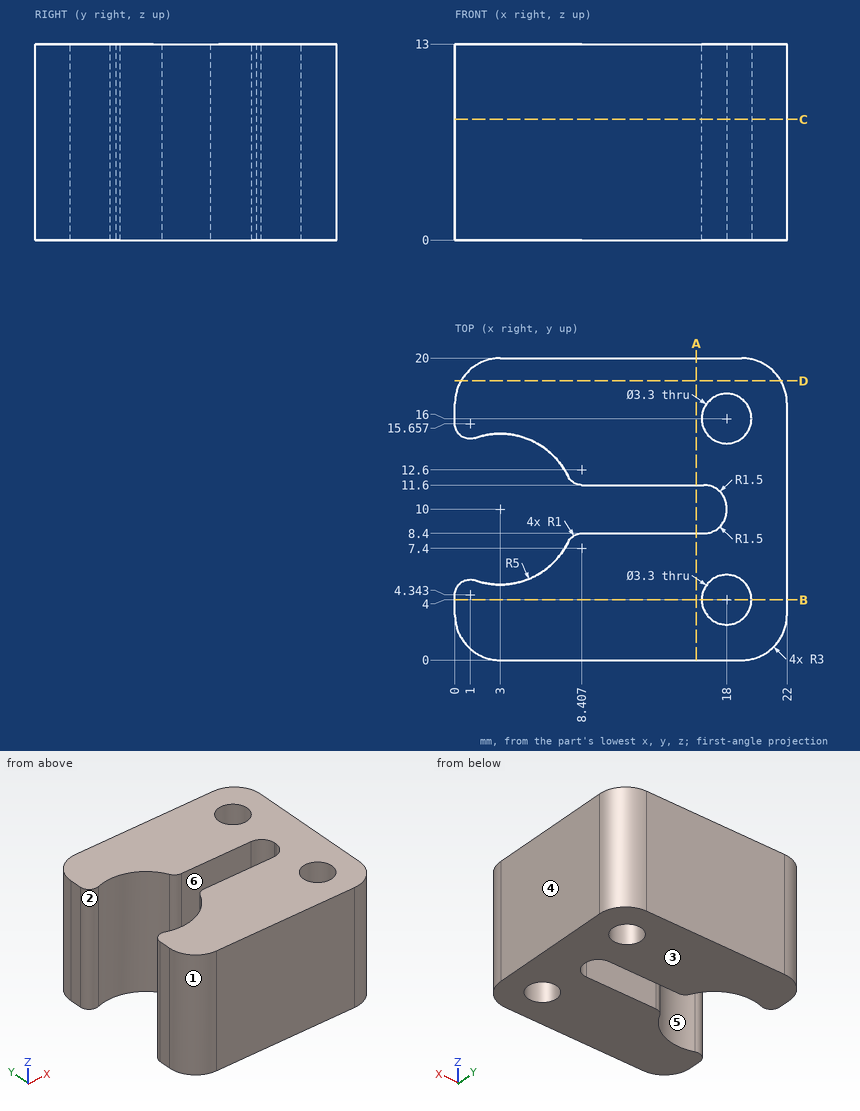
Here's the drawing with two shaded views (mm, measured from the low corner). I have some questions. A direction names the side the tool comes from. Give positions to 0.01 mm unless a question says otherwise; leave off trailing zeros. Loops run counter-clockwise (first coordinate to the right, second up) from the corner with the lowest first, then second, coordinate; pieces in that order, holes last. Notation, with made-up numbers: (-20, 68.5) - (21, 68.5) arc R37 cw to (21, 107.5) - close; hole circle Ø5 at (8, 79.25). An arc over 180 degrees is marked (long way). Answer in a Markdown table with one row per item. Add a question column.
Q1. If we section it at B-B (y = 4): List the corners of the cut face in (x, z) for me, plus the area to 3 significant figures.
Q2. For pin 1 (6 mm diameter, centred on y = 9.5, z = 6.5, fed in from -X); pin 2 (2.5 mm diameter, centred on x = 18, y = 16, fed in from +Z), each with a flat end and sliding along its axis, tell me the tip position at first contact or that it passes through.
Q3. Please list where these lines run through material, in increasing order: L1, parallel to Y at x = 14, z = 9.5; L2, parallel to Y at x = 4.75, z = 12.25 (1 decimal); L3, parallel to Y at x = 16.75, z = 10.5 (1 decimal). Write a range as from..to.
Q4. We'd pull the mould along X, two halves only. Please class the marked faces 1, 2 and 3: +X half, -X half, draft (parallel to the pull), parting line (faces both ways), or undercut.
Q5. If we section it at C-C (z = 8): List the corners of the cut face in (x, y) for me, plus the area to 3 significant figures.
Q6. Which directions (+Z, -Z, +X, -X, +Y, -Y) give clear straight access to the entire face, cutting with the end or side of a thin tool? Please do the marked faces 4, 5 and 6.
Q7. If we section it at D-D (y = 18.5): List the corners of the cut face in (x, z) for me.
Q8. If we section it at A-A (x = 16): List the corners of the cut face in (y, z) for me.
The answers:
| question | item | result |
|---|---|---|
| 1 | outline | (0, 0) - (16.35, 0) - (16.35, 13) - (0, 13) - close; (19.65, 0) - (22, 0) - (22, 13) - (19.65, 13) - close |
| 1 | area | 243 mm^2 |
| 2 | pin 1 | stops at x = 6.57 |
| 2 | pin 2 | passes through |
| 3 | L1 | y = 0..8.4, 11.6..20 |
| 3 | L2 | y = 0..5.3, 14.7..20 |
| 3 | L3 | y = 0..2.9, 5.1..8.4, 11.6..14.9, 17.1..20 |
| 4 | face 1 | -X half |
| 4 | face 2 | undercut |
| 4 | face 3 | draft |
| 5 | outline | (0, 3) arc R3 ccw to (3, 0) - (19, 0) arc R3 ccw to (22, 3) - (22, 17) arc R3 ccw to (19, 20) - (3, 20) arc R3 ccw to (0, 17) - (0, 15.66) arc R1 ccw to (1.33, 14.71) arc R5 cw to (7.51, 12.17) arc R1 ccw to (8.41, 11.6) - (16.5, 11.6) arc R1.5 cw to (18, 10.1) - (18, 9.9) arc R1.5 cw to (16.5, 8.4) - (8.41, 8.4) arc R1 ccw to (7.51, 7.83) arc R5 cw to (1.33, 5.29) arc R1 ccw to (0, 4.34) - close; hole circle Ø3.3 at (18, 4); hole circle Ø3.3 at (18, 16) |
| 5 | area | 315 mm^2 |
| 6 | face 4 | +Z, -Z, +X, +Y, -Y |
| 6 | face 5 | +Z, -Z |
| 6 | face 6 | +Z, -Z, -X |
| 7 | outline | (0.4, 0) - (21.6, 0) - (21.6, 13) - (0.4, 13) - close |
| 8 | outline | (0, 0) - (8.4, 0) - (8.4, 13) - (0, 13) - close; (11.6, 0) - (20, 0) - (20, 13) - (11.6, 13) - close |
